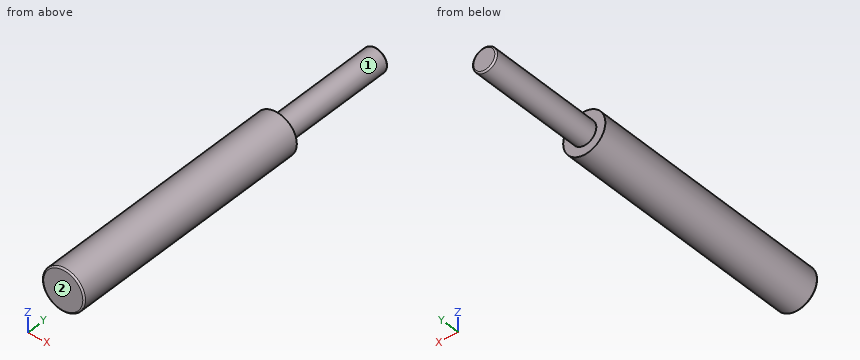
from build123d import *

# Parameters (mm, degrees)
SKETCH1_R           = 4
BOSS_EXTRUDE1_DEPTH = 40
SKETCH1_3_R         = 7
SKETCH1_3_R_2       = 4
BOSS_EXTRUDE2_DEPTH = 85
FILLET1_R           = 0.5


with BuildPart() as part:
    # Sketch1 → Boss-Extrude1 (new body)
    with BuildSketch(Plane(origin=(0, 0, 0), x_dir=(1, 0, 0), z_dir=(0, 1, 0))):
        Circle(SKETCH1_R)
    extrude(amount=BOSS_EXTRUDE1_DEPTH)

    # Sketch1_3 → Boss-Extrude2 (add)
    with BuildSketch(Plane(origin=(0, 0, 0), x_dir=(1, 0, 0), z_dir=(0, 1, 0))):
        Circle(SKETCH1_3_R)
        Circle(SKETCH1_3_R_2, mode=Mode.SUBTRACT)
        Circle(SKETCH1_3_R_2)
    extrude(amount=-BOSS_EXTRUDE2_DEPTH)

    # Fillet1
    fillet1_edges = [part.edges().sort_by_distance(p)[0] for p in [
        (-4, 40, 0),
        (-7, -85, 0),
    ]]
    fillet(fillet1_edges, radius=FILLET1_R)


solid = part.part
Could you check a few things on this model? Use its own coordinates, in mm. Face numbers are marked on the shaded views. A direction names the side the tool comes from. Round coordinates to 2 decimals unless told otherwise and drop trailing zeros. Order: outer loops, then holes, each group sorted by start corner. A loop starts at its lowest first (then second) coordinate and runs counter-clockwise, first axis right, second up. Notation, with made-up numbers: M 8,-26.5 L 14,-26.5 A17 cw 14,4.5 Z; hole C -32.75,44 d10. An arc over 180 degrees is marked long. One line per item, written item: value.
(1) I'm going to push flat-ended pins straight in: P1, Ø1, axis at y = -4.5, z = -4, coming from the -X side; P2, Ø4, axis at x = -1, y = -54.5, coming from the +Z side. Where does each tip first touch, or does it pass through?
Ans:
P1: stops at x = -6.06
P2: stops at z = 7
(2) Imagine slicing it at B-B (y = 2). Write out the boundary of the cut face in (x, z).
Ans:
outline: C 0,0 d8
(3) I need wall thicknesses on line 1 along X through (y, z) = (-5, 5.75); line 2 along Y through (x, z) = (1.5, -3.25); line 3 along Y through (x, z) = (1.5, -6). Which ranges of each line are inside material? Lowest first, please. Write a range as from..to.
Ans:
line 1: x = -3.99..3.99
line 2: y = -85..39.99
line 3: y = -85..0
(4) Imagine slicing it at C-C (y = -53). Write out the boundary of the cut face in (x, z).
Ans:
outline: C 0,0 d14
(5) Imagine slicing it at A-A (x = 0). Write out the boundary of the cut face in (y, z).
Ans:
outline: M -85,-6.5 A0.5 ccw -84.5,-7 L 0,-7 L 0,-4 L 39.5,-4 A0.5 ccw 40,-3.5 L 40,3.5 A0.5 ccw 39.5,4 L 0,4 L 0,7 L -84.5,7 A0.5 ccw -85,6.5 Z
(6) Which directions (+Z, -Z, +X, -X, +Y, -Y) give clear straight access to the entire face, cutting with the end or side of a thin tool? Please do the marked faces 1 and 2.
Ans:
face 1: +Y
face 2: +Z, -Z, +X, -X, -Y
